The model under review builds one solid part; all positions refer to its coordinate system, in mm. Face numbers are marked on the shaded views. Coordinates: 2 decimals unless noted, no trailing zeros. Loops run counter-clockwise (first coordinate to the right, second up) from the corner with the lowest first, then second, coordinate; pieces in that order, holes last. Notation, with made-up numbers: M 88,-15.75 L 97,-15.75 A17 ccw 97,-6.75 Z; hole C -38.5,24 d8. An arc over 180 degrees is marked long. Write item = value, one per line. Start each with the question number.
Q1. We need section A-A on z = 17. Give the boundary of the cut face in (x, y), and give its area (3 significant figures).
Q2. Clearance check with flat-ended pins moving along their axes: pin 1 Ø4 at (x, y) = (3, -1) entering from +Z; pin 2 Ø15.5 at (y, z) = (-11.5, 53.5) entering from -X; pin 3 Ø1 at (x, y) = (-32, -22) entering from +Z. State where each tip first meets the part, or that it passes through.
Q3. Wall thickness on probe 1 along Z at (x, y) = (8.5, 0); probe 2 along Z at (x, y) = (4.5, 11.5); probe 3 along X at (y, z) = (-36.5, 51): over which ranges is each line inside the solid? List them lowest first.
Q4. Mouldability with a two-part tool opening along X and no side actions: class the marked faces 1, 2, 3 and 4 as released by +X, released by -X, zero draft, split by the parting line, or undercut.
from build123d import *

# Parameters (mm, degrees)
F0_R      = 45.5235141672
F1_DEPTH  = 20
F2_DEPTH  = 50
F3_R      = 40
F4_W      = 12.5344563276
F4_H      = 31.0147441924
F5_DEPTH  = 100
F7_DEPTH  = 100
F8_R      = 2.5
F9_DEPTH  = 4
F10_R     = 2.5
F11_DEPTH = 4


with BuildPart() as f1:
    # F0 (on Top) → F1 (new body)
    with BuildSketch(Plane.XY):
        Circle(F0_R)
    extrude(amount=F1_DEPTH)

    # F2 (add): a face of the model
    f2_faces = [f1.faces().sort_by_distance(p)[0] for p in [
        (0, 0, 20),
    ]]
    extrude(f2_faces, amount=F2_DEPTH)

    # F3
    f3_edges = [f1.edges().sort_by_distance(p)[0] for p in [
        (-45.523514, 0, 70),
    ]]
    fillet(f3_edges, radius=F3_R)

    # F4 (on Front) → F5 (cut)
    with BuildSketch(Plane.XZ):
        with Locations((-0.0651595183, 54.6367447823)):
            Rectangle(F4_W, F4_H)
    extrude(amount=-F5_DEPTH, mode=Mode.SUBTRACT)

    # F6 (on face) → F7 (cut)
    with BuildSketch(Plane(origin=(0, 0, 0), x_dir=(-1, 0, 0), z_dir=(0, 1, 0))):
        with BuildLine():
            ThreePointArc((-5.5235141672, 70), (-5.8628036122, 69.9985610075), (-6.2020686455, 69.9942441336))
            Line((-6.2020686455, 69.9942441336), (-6.2020686455, 39.1293726861))
            Line((-6.2020686455, 39.1293726861), (6.3323876821, 39.1293726861))
            Line((6.3323876821, 39.1293726861), (6.3323876821, 69.9918207092))
            add(Edge.make_bspline(
                [(6.3323876821, 69.9918207092), (6.1301968719, 69.9959102152), (5.927978494, 69.9986367384), (5.7257463298, 70), (5.5235141672, 70)],
                knots=[0.6079316836, 0.6079316836, 0.6079316836, 0.6079316836, 0.6079316836, 1, 1, 1, 1, 1], degree=4))
            Line((5.5235141672, 70), (-5.5235141672, 70))
        make_face()
    extrude(amount=-F7_DEPTH, mode=Mode.SUBTRACT)

    # F8 (on face) → F9 (cut)
    with BuildSketch(Plane.YZ.offset(-6.3323876821)):
        with Locations((0, 46.6293726861)):
            Circle(F8_R)
    extrude(amount=-F9_DEPTH, mode=Mode.SUBTRACT)

    # F10 (on face) → F11 (cut)
    with BuildSketch(Plane(origin=(6.2020686455, 0, 0), x_dir=(0, -1, 0), z_dir=(-1, 0, 0))):
        with Locations((0, 46.6293726861)):
            Circle(F10_R)
    extrude(amount=-F11_DEPTH, mode=Mode.SUBTRACT)


solid = f1.part
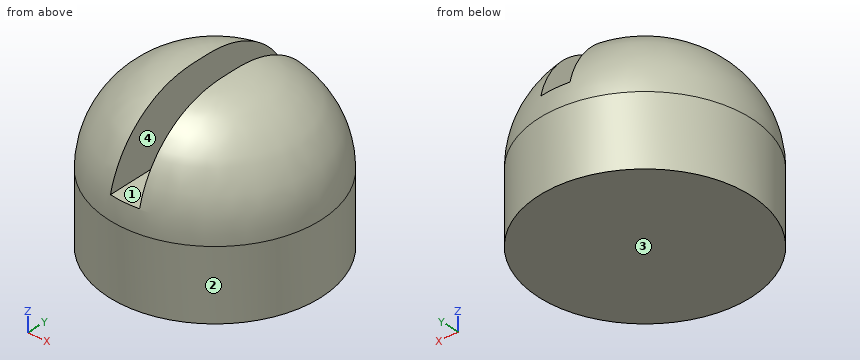
Returned:
q1.outline = C 0,0 d91.05
q1.area = 6,510 mm^2
q2.pin_1 = 39.13
q2.pin_2 = -41.16
q2.pin_3 = 52.88
q3.probe_1 = 0 to 44.13, 49.13 to 69.89
q3.probe_2 = 0 to 39.13
q3.probe_3 = -15.28 to -6.33, 6.2 to 15.28
q4.face_1 = undercut
q4.face_2 = split by the parting line
q4.face_3 = zero draft
q4.face_4 = undercut
